Job drawing, mm, ordinate dimensions from the low corner. One solid piece. Coordinates: 2 decimals unless noted, no trailing zeros. Loops run counter-clockwise (first coordinate to the right, second up) from the corner with the lowest first, then second, coordinate; pieces in that order, holes last. Notation, with made-up numbers: M 52,-6 L 111,-6 A11 ccw 111,6 Z; hole C 12,-28 d9. An arc over 180 degrees is marked long. Answer as a JSON object with one key per item and string values. Group by question number.
1. Saw through at A-A on y = 10.5. Write the cut outline in (x, z).
2. Drop a flat-ended pin along its axis: pin 1 Ø17.5 at (x, z) = (14, 79.5) entering from +Y. Give the stop position or say it passes through.
3. Saw through at B-B on x = 19. Write the cut outline in (y, z).
4. Drill centre lines: L1, parallel to Y at x = 6.25, z = 59.5; L2, parallel to X at y = 36, z = 48.5; L3, parallel to Y at x = 11, z = 83.5. Where is each one in solid material? Low to high.
5. Saw through at C-C on z = 64. Write the cut outline in (x, y).
6. Saw through at D-D on z = 109. Write the cut outline in (x, y), then the cut area to 3 significant figures.
7. Mould opens along X. For the marked faces 1, 2, 3 and 4 say: released by +X, released by -X, zero draft, split by the parting line, or undercut.
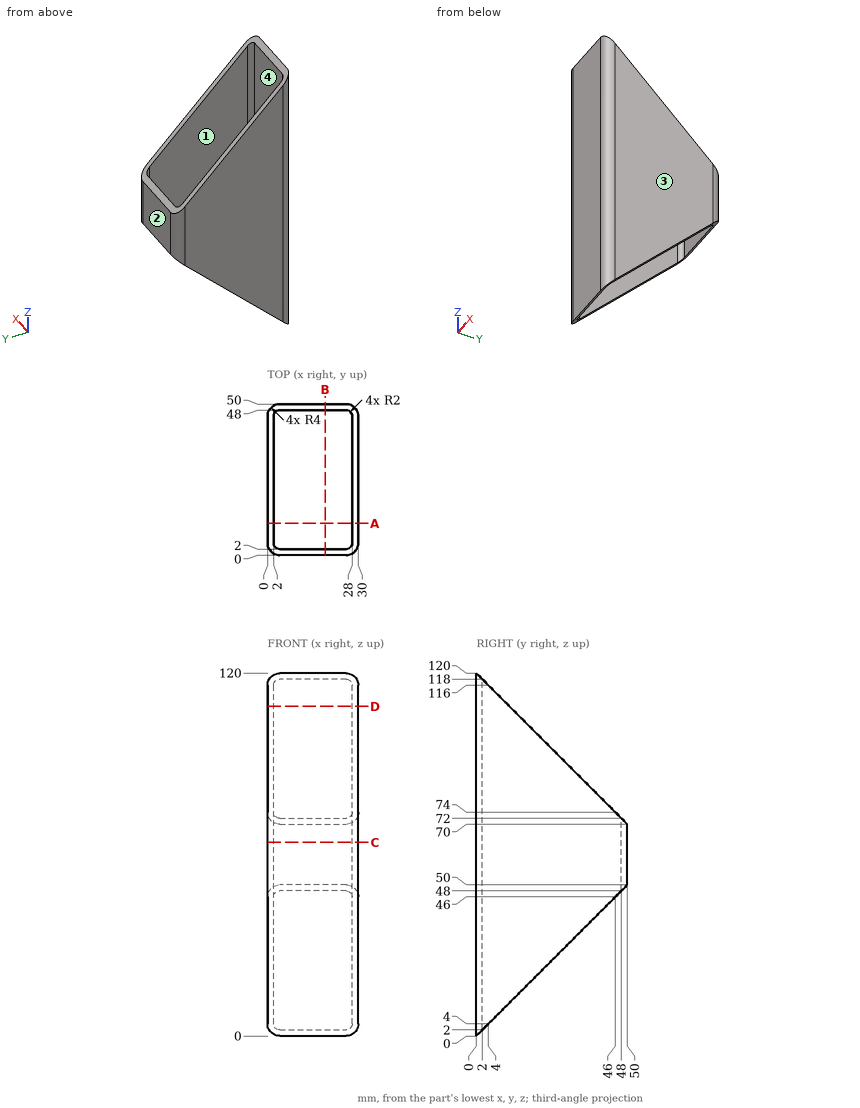
Outcome:
{
 "1": {"outline": "M 0,10.5 L 2,10.5 L 2,109.5 L 0,109.5 Z; M 28,10.5 L 30,10.5 L 30,109.5 L 28,109.5 Z"},
 "2": {"pin 1": "stops at y = 49.25"},
 "3": {"outline": "M 0,0 L 2,2 L 2,118 L 0,120 Z; M 48,48 L 50,50 L 50,70 L 48,72 Z"},
 "4": {"L1": "y = 0 to 2, 48 to 50", "L2": "x = 0 to 2, 28 to 30", "L3": "y = 0 to 2"},
 "5": {"outline": "M 0,4 A4 ccw 4,0 L 26,0 A4 ccw 30,4 L 30,46 A4 ccw 26,50 L 4,50 A4 ccw 0,46 Z; hole M 2,4 A2 ccw 4,2 L 26,2 A2 ccw 28,4 L 28,46 A2 ccw 26,48 L 4,48 A2 ccw 2,46 Z"},
 "6": {"outline": "M 0,4 A4 ccw 4,0 L 26,0 A4 ccw 30,4 L 30,11 L 28,11 L 28,4 A2 cw 26,2 L 4,2 A2 cw 2,4 L 2,11 L 0,11 Z", "area": "90.8 mm²"},
 "7": {"face 1": "undercut", "face 2": "zero draft", "face 3": "released by +X", "face 4": "undercut"}
}
